The drawing under review shows one solid part. Ordinate dimensions are in mm from its lowest x, y, z. A direction names the side the tool comes from. Round coordinates to 2 decimals unless told otherwise and drop trailing zeros. Order: outer loops, then holes, each group sorted by start corner. A loop starts at its lowest first (then second) coordinate and runs counter-clockwise, first axis right, second up. Notation, with made-up numbers: (32, 75.25) -> (81, 75.25) arc R13 ccw to (81, 87.25) -> close; hole circle Ø6 at (-37.75, -12). An arc over 180 degrees is marked (long way). Use a Markdown table: item, result. Add a question column.
1) Consider section B-B (z = 5.75). State the section outline as (x, y) points (1 decimal), plus the area to 3 significant figures.
2) Clearance check with a flat-ended pin moving along its axis: P1, Ø1, axis at x = 1, z = 5, coming from the +Y side (1 decimal). State where the tip first meets the part, or that it passes through.
3) Consider section C-C (y = 4). State the section outline as (x, z) points (1 decimal).
4) Machinability: for the marked faces 1 and 2, which of the approach directions +Z, -Z, +X, -X, +Y, -Y give a long, thin tool a straight path to every point of the face, cutting with its end or side? Answer none if there is none.
5) Consider section D-D (x = 0.5). State the section outline as (y, z) points.
6) Draft analysis for pull direction Y (two halves, no side actions). For the marked faces 3, 4, 5 and 6, state which applies: pulls with the +Y half, pulls with the -Y half, needs draft (parallel to the pull), parting line crosses it, or undercut.
7) Wall thickness on line 1 along Y through (x, z) = (2.63, 1.5) (1 decimal); line 2 along X through (y, z) = (3, 9.5) (1 decimal); line 3 along Z through (x, y) = (1.3, 1.35): over which ranges is each line inside the solid? List them lowest first. Write a range as [from, to].
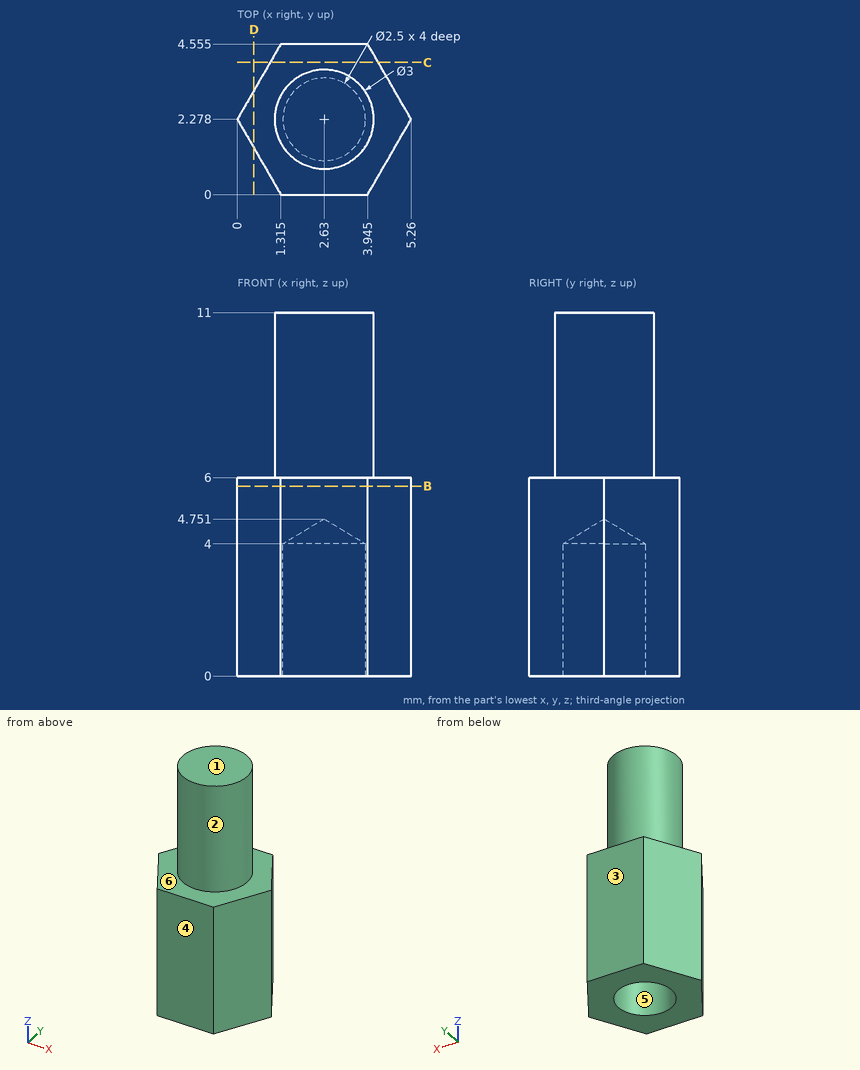
Results list:
| question | item | result |
|---|---|---|
| 1 | outline | (0, 2.3) -> (1.3, 0) -> (3.9, 0) -> (5.3, 2.3) -> (3.9, 4.6) -> (1.3, 4.6) -> close |
| 1 | area | 18.0 mm2 |
| 2 | P1 | y = 4.6 |
| 3 | outline | (1, 0) -> (4.3, 0) -> (4.3, 6) -> (1, 6) -> close |
| 4 | face 1 | +Z, +X, -X, +Y, -Y |
| 4 | face 2 | +Z |
| 5 | outline | (1.41, 0) -> (3.14, 0) -> (3.14, 6) -> (1.41, 6) -> close |
| 6 | face 3 | pulls with the +Y half |
| 6 | face 4 | pulls with the -Y half |
| 6 | face 5 | undercut |
| 6 | face 6 | needs draft |
| 7 | line 1 | [0, 1], [3.5, 4.6] |
| 7 | line 2 | [1.3, 3.9] |
| 7 | line 3 | [0, 6] |
